from build123d import *

# Parameters (mm, degrees)
SKETCH1_R           = 18
BOSS_EXTRUDE1_DEPTH = 82.6
SKETCH3_R           = 1.5
CUT_EXTRUDE1_DEPTH  = 5
SKETCH2_R           = 4
BOSS_EXTRUDE3_DEPTH = 15


with BuildPart() as part:
    # Sketch1 → Boss-Extrude1 (new body)
    with BuildSketch(Plane.XY):
        with Locations(Location((0, 0, 0), (0, 0, 180))):
            Circle(SKETCH1_R)
    extrude(amount=BOSS_EXTRUDE1_DEPTH)

    # Sketch3 → Cut-Extrude1 (cut)
    with BuildSketch(Plane(origin=(0, 0, 0), x_dir=(-1, 0, 0), z_dir=(0, 0, -1))):
        with Locations((0, 14)):
            Circle(SKETCH3_R)
        with Locations((14, 0)):
            Circle(SKETCH3_R)
        with Locations((0, -14)):
            Circle(SKETCH3_R)
        with Locations((-14, 0)):
            Circle(SKETCH3_R)
    extrude(amount=-CUT_EXTRUDE1_DEPTH, mode=Mode.SUBTRACT)

    # Sketch2 → Boss-Extrude3 (add)
    with BuildSketch(Plane(origin=(0, 0, 0), x_dir=(-1, 0, 0), z_dir=(0, 0, -1))):
        with Locations(Location((0, 0, 0), (0, 0, 180))):
            Circle(SKETCH2_R)
    extrude(amount=BOSS_EXTRUDE3_DEPTH)


solid = part.part
Can you work these out from the model? Positions are in its coordinate system, mm. A direction names the side the tool comes from. Coordinates: 2 decimals unless noted, no trailing zeros. Loops run counter-clockwise (first coordinate to the right, second up) from the corner with the lowest first, then second, coordinate; pieces in that order, holes last. Notation, with made-up numbers: M -33,61.25 L 4,61.25 A19 cw 4,90.25 Z; hole C 44.25,17.5 d5. An arc over 180 degrees is marked long. Return JSON: item names as keys, results as strings. Group by question number.
Item 1: On a 3-axis mill with a long thin cutter (end or side, diameter ignored), from which of +Z, -Z, +X, -X, +Y, -Y can I reach the whole of each face in a straight line? I mean faces 1 (the cylindrical face through (-12.5, 0.07, 2.46)), 2 (the cylindrical face through (13.267, -12.165, 40.722)). Say none if no direction works.
Item 2: Imagine slicing it at C-C (z = 77.5). Please give me the cut outline in (x, y), and give its area (3 significant figures).
Item 3: I'm going to push flat-ended pins straight in: pin 1 Ø3 at (x, z) = (7, 28.5) entering from -Y; pin 2 Ø4 at (x, y) = (-14, 0) entering from -Z; pin 3 Ø2.5 at (x, y) = (0, 14) entering from -Z. Where does each tip first touch, or does it pass through?
Item 4: Thinking about a two-plate mould opening in Y: for faces 3 (the cylindrical face through (-0.867, 3.905, -7.395)), 4 (the cylindrical face through (0.325, -15.464, 2.465)), 5 (the flat face through (0, 0, -15)), which applies, released by +Y, released by -Y, zero draft, split by the parting line, or undercut?
Item 5: Imagine slicing it at D-D (y = 8.5). Please give me the cut outline in (x, z), and give its area (3 significant figures).
Item 6: If I drill on L1, parallel to Y at x = 0, z = 1; L2, parallel to Z at x = -4, y = -11; L3, parallel to Z at x = 13, y = -1, over which ranges is the centre line in solid material (lowest first)? Write a range as from..to.
Item 7: Imagine slicing it at A-A (x = 14). Please give me the cut outline in (y, z).
Verdict:
{
 "1": {"face 1": "-Z", "face 2": "+Z, -Z"},
 "2": {"outline": "C 0,0 d36", "area": "1,020 mm^2"},
 "3": {"pin 1": "stops at y = -17.14", "pin 2": "stops at z = 0", "pin 3": "stops at z = 5"},
 "4": {"face 3": "split by the parting line", "face 4": "undercut", "face 5": "zero draft"},
 "5": {"outline": "M -15.87,0 L 15.87,0 L 15.87,82.6 L -15.87,82.6 Z", "area": "2,620 mm^2"},
 "6": {"L1": "y = -18..-15.5, -12.5..12.5, 15.5..18", "L2": "z = 0..82.6", "L3": "z = 5..82.6"},
 "7": {"outline": "M -11.31,0 L -1.5,0 L -1.5,5 L 1.5,5 L 1.5,0 L 11.31,0 L 11.31,82.6 L -11.31,82.6 Z"}
}
